Build history of the part. All positions in model axes, mm. A direction names the side the tool comes from. Give positions to 0.01 mm unless a question says otherwise; leave off trailing zeros. Order: outer loops, then holes, each group sorted by start corner. A loop starts at its lowest first (then second) coordinate and runs counter-clockwise, first axis right, second up. Notation, with made-up numbers: (84, 45.5) -> (94, 45.5) arc R29 cw to (94, 65.5) -> close; hole circle Ø8 at (5.25, 29). An arc over 180 degrees is marked (long way). One line per item, written item: value. Start each with the question number.
(1) Saw through at C-C on x = 47. Give the cut face in (y, z), plus the area to 3 significant figures.
(2) Pin check, flat tips, straight feed: pin 1 (12 mm diameter, centred on y = 94.5, z = 136.5, fed in from +X); pin 2 (3 mm diameter, centred on x = 73.5, y = 109.5, fed in from +Z); pin 3 (4 mm diameter, centred on y = 72.5, z = -162.5, fed in from +X). Stop position of each tip, or through.
(3) Saw through at A-A on x = 173. Give the cut face in (y, z).
(4) Saw through at B-B on z = 73.5. Give the cut face in (x, y), plus the area to 3 significant figures.
(5) Which spindle directions (+Z, -Z, +X, -X, +Y, -Y) get a long thin tool onto all of the face, cutting with end or side? Do faces 4 (the cylindrical face through (142.457, 0.986, -92.768)), 5 (the flat face through (174, 0, 29)), 6 (the flat face through (152, 2, -103)). Say none if no direction does.
(6) Probe line 1 (Y direction, x = 191, z = -38); line 2 (Z direction, x = 161.5, y = 128.5); line 3 (Z direction, x = 40.5, y = 116). List the from-to ranges inside material, lowest first.
(7) Saw through at D-D on y = 192.5. Give the cut face in (x, z).
(8) Two-plate mould, pull along Z, no slides. Class faces 1 (the flat face through (97.565, 0.986, 157.428)), 2 (the flat face through (174, 208, 29)), 3 (the cylindrical face through (204.956, 102.544, 4.227)): +Z half, -Z half, draft (parallel to the pull), parting line (faces both ways), or undercut.
```python
from build123d import *

# Parameters (mm, degrees)
BOSS_EXTRUDE1_DEPTH = 208
BOSS_EXTRUDE2_DEPTH = 2


with BuildPart() as part:
    # Sketch1 → Boss-Extrude1 (new body)
    with BuildSketch(Plane(origin=(0, 0, 0), x_dir=(1, 0, 0), z_dir=(0, 1, 0))):
        with BuildLine():
            Line((20, 204.022057631), (20, 198.997487421))
            ThreePointArc((20, 198.997487421), (200, 0), (20, -198.997487421))
            Line((20, -198.997487421), (20, -204.022057631))
            ThreePointArc((20, -204.022057631), (205, 0), (20, 204.022057631))
        make_face()
    extrude(amount=BOSS_EXTRUDE1_DEPTH)

    # Sketch2 → Boss-Extrude2 (add)
    with BuildSketch(Plane(origin=(0, 0, 0), x_dir=(1, 0, 0), z_dir=(0, 1, 0))):
        with BuildLine():
            Line((105.356537529, -170), (89.553056899, -144.5))
            ThreePointArc((89.553056899, -144.5), (141.892609151, -93.629522418), (168.076619433, -25.5))
            Line((168.076619433, -25.5), (197.737199333, -30))
            ThreePointArc((197.737199333, -30), (166.932481354, -110.152379315), (105.356537529, -170))
        make_face()
        with BuildLine():
            Line((197.737199333, 30), (168.076619433, 25.5))
            ThreePointArc((168.076619433, 25.5), (141.892609151, 93.629522418), (89.553056899, 144.5))
            Line((89.553056899, 144.5), (105.356537529, 170))
            ThreePointArc((105.356537529, 170), (166.932481354, 110.152379315), (197.737199333, 30))
        make_face()
    boss_extrude2 = extrude(amount=BOSS_EXTRUDE2_DEPTH)

    # Mirror1: Boss-Extrude2 across plane
    add(boss_extrude2.mirror(Plane.ZX.offset(104)))


solid = part.part
```
Results below:
1. outline: (0, -199.54) -> (208, -199.54) -> (208, -194.4) -> (0, -194.4) -> close; (0, 194.4) -> (208, 194.4) -> (208, 199.54) -> (0, 199.54) -> close
1. area: 2,140 mm²
2. pin 1: stops at x = 158.1
2. pin 2: stops at z = 191.94
2. pin 3: stops at x = 127.53
3. outline: (0, -109.98) -> (208, -109.98) -> (208, -26.25) -> (206, -26.25) -> (206, -100.35) -> (2, -100.35) -> (2, -26.25) -> (0, -26.25) -> close; (0, 26.25) -> (2, 26.25) -> (2, 100.35) -> (206, 100.35) -> (206, 26.25) -> (208, 26.25) -> (208, 109.98) -> (0, 109.98) -> close
4. outline: (153.29, 0) -> (191.37, 0) -> (191.37, 208) -> (153.29, 208) -> (153.29, 206) -> (186, 206) -> (186, 2) -> (153.29, 2) -> close
4. area: 1,250 mm²
5. face 4: -X, +Y, -Y
5. face 5: +Z, -Z, +X, -X, -Y
5. face 6: -X
6. line 1: y = 0 to 2, 206 to 208
6. line 2: z = -126.26 to -117.97, 117.97 to 126.26
6. line 3: z = -200.96 to -195.86, 195.86 to 200.96
7. outline: (20, -204.02) arc R205 ccw to (20, 204.02) -> (20, 199) arc R200 cw to (20, -199) -> close
8. face 1: undercut
8. face 2: draft
8. face 3: parting line
